from build123d import *

# Parameters (mm, degrees)
SKETCH1_R           = 15
BOSS_EXTRUDE1_DEPTH = 100
SKETCH3_W           = 70
SKETCH3_H           = 73.742288546
CUT_EXTRUDE1_DEPTH  = 50
CUT_EXTRUDE2_DEPTH  = 20


with BuildPart() as part:
    # Sketch1 → Boss-Extrude1 (new body)
    with BuildSketch(Plane.XY):
        with BuildLine():
            Line((-49.633171283, 65.600501081), (-49.633171283, -4.399498919))
            Line((-49.633171283, -4.399498919), (80.366828717, -4.399498919))
            Line((80.366828717, -4.399498919), (60.366828717, 14.358212535))
            Line((60.366828717, 14.358212535), (30.366828717, 14.358212535))
            Line((30.366828717, 14.358212535), (-7.909440204, 77.292300062))
            ThreePointArc((-7.909440204, 77.292300062), (-33.204252353, 87.265956872), (-49.633171283, 65.600501081))
        make_face()
        with Locations((-27.133171283, 65.600501081)):
            Circle(SKETCH1_R, mode=Mode.SUBTRACT)
    extrude(amount=-BOSS_EXTRUDE1_DEPTH)

    # Sketch3 → Cut-Extrude1 (cut, symmetric)
    with BuildSketch(Plane(origin=(0, 0, 0), x_dir=(0, 0, -1), z_dir=(1, 0, 0))):
        with Locations((50, 51.229356808)):
            Rectangle(SKETCH3_W, SKETCH3_H)
    extrude(amount=CUT_EXTRUDE1_DEPTH, both=True, mode=Mode.SUBTRACT)

    # Sketch4 → Cut-Extrude2 (cut, symmetric)
    with BuildSketch(Plane(origin=(0, 14.358212535, 0), x_dir=(1, 0, 0), z_dir=(0, 1, 0))):
        with BuildLine():
            Line((30.366828717, 67.683852826), (82.708182872, 67.683852826))
            Line((82.708182872, 67.683852826), (82.708182872, 27.683852826))
            Line((82.708182872, 27.683852826), (30.366828717, 27.683852826))
            ThreePointArc((30.366828717, 27.683852826), (10.366828717, 47.683852826), (30.366828717, 67.683852826))
        make_face()
    extrude(amount=CUT_EXTRUDE2_DEPTH, both=True, mode=Mode.SUBTRACT)


solid = part.part
Can you work these out from the model? Positions are in its coordinate system, mm. A direction names the side the tool comes from. Coordinates: 2 decimals unless noted, no trailing zeros. Order: outer loops, then holes, each group sorted by start corner. A loop starts at its lowest first (then second) coordinate and runs counter-clockwise, first axis right, second up. Notation, with made-up numbers: (-31.75, 35.5) - (9.25, 35.5) arc R9 cw to (9.25, 49.5) - close; hole circle Ø9 at (-25, 4). An arc over 180 degrees is marked (long way). Answer as a JSON object with one key per item and string values. Group by question number.
Q1. Will this pin go through, and if not, where does the flat tip stop? P1, Ø5.5, axis at x = 65, y = 9, coming from the +Z side.
Q2. Imagine slicing it at B-B (x = 49.5). Please give me the cut outline in (y, z).
Q3. Imagine slicing it at C-C (y = 70.5). Please give me the cut outline in (x, z), and give its area (3 significant figures).
Q4. I need wall thicknesses on line 1 (Z direction, x = -2, y = 30); line 2 (Y direction, x = 17, z = -16.5); line 3 (Y direction, x = -30.5, z = -11.5). Which ranges of each line are inside material? Lowest first, please. Write a range as from..to.
Q5. We'd pull the mould along Z, two halves only. Please class faces 4 (the face through (49, 5, -67.684)), 5 (the face through (0, 32, 0)), 6 (the face through (-42.12, 66.26, -92.4)): +Z half, -Z half, draft (parallel to the pull), parting line (faces both ways), or undercut.
Q6. On a 3-axis mill with a long thin cutter (end or side, diameter ignored), from which of +Z, -Z, +X, -X, +Y, -Y can I reach the whole of each face in a straight line? I mean faces 1 (the face through (-18, 43, -15)), 2 (the face through (0, -4.399, -49)), 3 (the face through (50, 5, -27.684)). Say none if no direction works.
Q7. Imagine slicing it at A-A (z = -8.5). Please give me the cut outline in (x, y).
Q8. Imagine slicing it at D-D (x = -34.5). Please give me the cut outline in (y, z), and give its area (3 significant figures).
Determined:
{
 "1": {"P1": "stops at z = 0"},
 "2": {"outline": "(-4.4, -100) - (14.36, -100) - (14.36, -67.68) - (-4.4, -67.68) - close; (-4.4, -27.68) - (14.36, -27.68) - (14.36, 0) - (-4.4, 0) - close"},
 "3": {"outline": "(-49.09, -100) - (-41.31, -100) - (-41.31, -85) - (-49.09, -85) - close; (-49.09, -15) - (-41.31, -15) - (-41.31, 0) - (-49.09, 0) - close; (-12.96, -100) - (-3.78, -100) - (-3.78, -85) - (-12.96, -85) - close; (-12.96, -15) - (-3.78, -15) - (-3.78, 0) - (-12.96, 0) - close", "area": "509 mm2"},
 "4": {"line 1": "z = -100..-85, -15..0", "line 2": "y = -4.4..14.36", "line 3": "y = -4.4..50.98, 80.22..87.85"},
 "5": {"face 4": "undercut", "face 5": "+Z half", "face 6": "draft"},
 "6": {"face 1": "+X, -X, +Y", "face 2": "+Z, -Z, +X, -X, -Y", "face 3": "+X, +Y, -Y"},
 "7": {"outline": "(-49.63, -4.4) - (80.37, -4.4) - (60.37, 14.36) - (30.37, 14.36) - (-7.91, 77.29) arc R22.5 ccw to (-49.63, 65.6) - close; hole circle Ø30 at (-27.13, 65.6)"},
 "8": {"outline": "(-4.4, -100) - (52.53, -100) - (52.53, -85) - (14.36, -85) - (14.36, -15) - (52.53, -15) - (52.53, 0) - (-4.4, 0) - close; (78.67, -100) - (86.86, -100) - (86.86, -85) - (78.67, -85) - close; (78.67, -15) - (86.86, -15) - (86.86, 0) - (78.67, 0) - close", "area": "3,270 mm2"}
}
